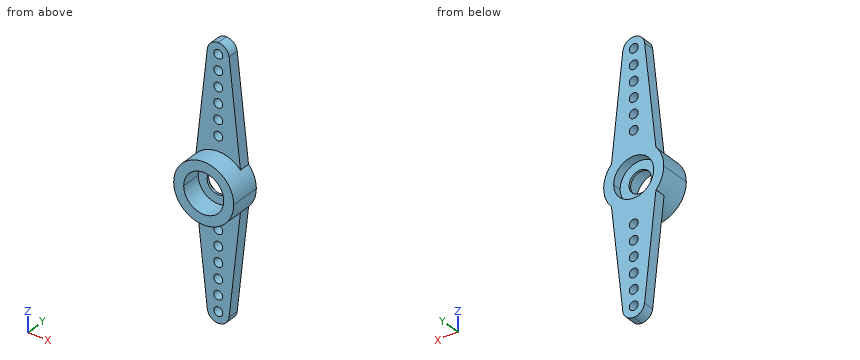
from build123d import *

# Parameters (mm, degrees)
SKETCH1_R               = 3.429
SKETCH1_R_2             = 2.286
BOSS_EXTRUDE1_DEPTH     = 3.556
BOSS_EXTRUDE2_DEPTH     = 1.27
BOSS_EXTRUDE3_START     = -1.016
SKETCH2_3_R             = 2.286
SKETCH2_3_R_2           = 1.27
BOSS_EXTRUDE3_DEPTH     = 0.254
SKETCH3_R               = 0.508
CUT_EXTRUDE1_DEPTH      = 17.020635974
LPATTERN1_COUNT         = 6
LPATTERN1_PITCH         = 1.778
SKETCH4_W               = 4.326879353
SKETCH4_H               = 6.724216597
CUT_EXTRUDE2_DEPTH      = 17.020635974
CUT_EXTRUDE2_DEPTH_BACK = 17.020635974


with BuildPart() as part:
    # Sketch1 → Boss-Extrude1 (new body)
    with BuildSketch(Plane(origin=(0, 0, 0), x_dir=(1, 0, 0), z_dir=(0, 1, 0))):
        with Locations(Location((0, 0, 0), (0, 0, 270))):
            Circle(SKETCH1_R)
        with Locations(Location((0, 0, 0), (0, 0, 270))):
            Circle(SKETCH1_R_2, mode=Mode.SUBTRACT)
    extrude(amount=BOSS_EXTRUDE1_DEPTH)

    # Sketch2 → Boss-Extrude2 (add)
    with BuildSketch(Plane(origin=(0, 3.556, 0), x_dir=(1, 0, 0), z_dir=(0, 1, 0))):
        with BuildLine():
            ThreePointArc((-2.54, 2.303571358), (-1.389081498, 3.135042837), (0, 3.429))
            Line((0, 3.429), (0, 15.24))
            ThreePointArc((0, 15.24), (-0.835660201, 14.92028345), (-1.244511661, 14.124427226))
            Line((-1.244511661, 14.124427226), (-2.54, 2.303571358))
        make_face()
        with BuildLine():
            Line((0, 15.24), (0, 3.429))
            ThreePointArc((0, 3.429), (1.389081498, 3.135042837), (2.54, 2.303571358))
            Line((2.54, 2.303571358), (1.244511661, 14.124427226))
            ThreePointArc((1.244511661, 14.124427226), (0.835660201, 14.92028345), (0, 15.24))
        make_face()
    extrude(amount=-BOSS_EXTRUDE2_DEPTH)

    # Sketch2_3 → Boss-Extrude3 (add)
    with BuildSketch(Plane(origin=(0, 3.556, 0), x_dir=(1, 0, 0), z_dir=(0, 1, 0)).offset(BOSS_EXTRUDE3_START)):
        with Locations(Location((0, 0, 0), (0, 0, 270))):
            Circle(SKETCH2_3_R)
        with Locations(Location((0, 0, 0), (0, 0, 270))):
            Circle(SKETCH2_3_R_2, mode=Mode.SUBTRACT)
    extrude(amount=-BOSS_EXTRUDE3_DEPTH)

    # Sketch3 → Cut-Extrude1 (cut, through all)
    with BuildSketch(Plane(origin=(0, 3.556, 0), x_dir=(1, 0, 0), z_dir=(0, 1, 0))):
        with Locations(Location((0, 5.08, 0), (0, 0, 270))):
            Circle(SKETCH3_R)
    cut_extrude1 = extrude(amount=-CUT_EXTRUDE1_DEPTH, mode=Mode.SUBTRACT)

    # LPattern1: Cut-Extrude1 ×6
    with Locations(*[(0, 0, -i * LPATTERN1_PITCH) for i in range(1, LPATTERN1_COUNT)]):
        add(cut_extrude1, mode=Mode.SUBTRACT)

    # Sketch4 → Cut-Extrude2 (cut, two sides)
    with BuildSketch(Plane(origin=(0, 0, 0), x_dir=(0, 0, -1), z_dir=(1, 0, 0))) as cut_extrude2_sk:
        with Locations((-2.163439677, 3.362108299)):
            Rectangle(SKETCH4_W, SKETCH4_H)
    extrude(amount=CUT_EXTRUDE2_DEPTH, mode=Mode.SUBTRACT)
    extrude(cut_extrude2_sk.sketch, amount=-CUT_EXTRUDE2_DEPTH_BACK, mode=Mode.SUBTRACT)

    # Mirror1: part across plane


with BuildPart() as part_1:
    add(part.part)
    add(part.part.mirror(Plane.XY))


solid = part_1.part
Geometry: final body of the model. Coordinates: model frame, mm. Round coordinates to 2 decimals unless told otherwise and drop trailing zeros. Order: outer loops, then holes, each group sorted by start corner. A loop starts at its lowest first (then second) coordinate and runs counter-clockwise, first axis right, second up. Notation, with made-up numbers: (11.25, 51.5) -> (51.25, 51.5) arc R34 ccw to (51.25, 87.5) -> close; hole circle Ø11 at (26.25, 8). An arc over 180 degrees is marked (long way). Put each result on its own line as item: value. Start each with the question number.
Q1. Section C-C on x = 2. Return the cut outline in (y, z).
Q2. Section D-D on z = -2. Return the cut outline in (x, y), and give its area (3 significant figures).
Q3. Line query: probe 1 along Y at (x, z) = (0.5, -3.5); probe 2 along Z at (x, y) = (2, 1.05); probe 3 along Z at (x, y) = (0.5, 0.45). Output: solid intervals per line, ascending.
Q4. Section B-B on y = 2. Return the cut outline in (x, z).
Q5. First-contact query: pin 1 (2.5 mm diameter, centred on x = -1, z = 6, fed in from -Y); pin 2 (1.5 mm diameter, centred on y = 2, z = -4.5, fed in from +X). Flat tips, straight axial feed; report the tip coordinate or a pass-through.
Q6. Section A-A on z = 5. Return the cut outline in (x, y), and give its area (3 significant figures).
Ans:
1. outline: (0, -2.79) -> (2.29, -2.79) -> (2.29, -7.23) -> (3.56, -7.23) -> (3.56, -1.11) -> (2.54, -1.11) -> (2.54, 1.11) -> (3.56, 1.11) -> (3.56, 7.23) -> (2.29, 7.23) -> (2.29, 2.79) -> (0, 2.79) -> (0, 1.11) -> (2.29, 1.11) -> (2.29, -1.11) -> (0, -1.11) -> close
2. outline: (-2.79, 0) -> (-1.11, 0) -> (-1.11, 2.29) -> (1.11, 2.29) -> (1.11, 0) -> (2.79, 0) -> (2.79, 3.56) -> (1.11, 3.56) -> (1.11, 2.54) -> (-1.11, 2.54) -> (-1.11, 3.56) -> (-2.79, 3.56) -> close
2. area: 12.5 mm2
3. probe 1: y = 2.29 to 3.56
3. probe 2: z = -2.79 to -1.11, 1.11 to 2.79
3. probe 3: z = -3.39 to -2.23, 2.23 to 3.39
4. outline: circle Ø6.86 at (0, 0); hole circle Ø4.57 at (0, 0)
5. pin 1: stops at y = 2.29
5. pin 2: stops at x = 2.38
6. outline: (-2.24, 2.29) -> (-0.5, 2.29) -> (-0.5, 3.56) -> (-2.24, 3.56) -> close; (0.5, 2.29) -> (2.24, 2.29) -> (2.24, 3.56) -> (0.5, 3.56) -> close
6. area: 4.43 mm2
